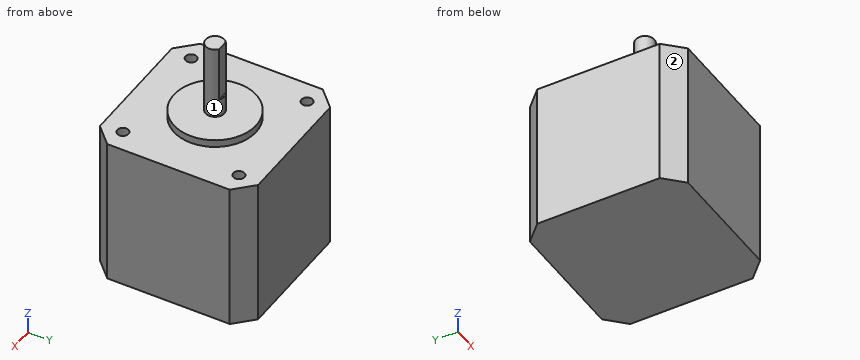
from build123d import *

# Parameters (mm, degrees)
F0_W      = 42.291
F0_H      = 42.291
F1_DEPTH  = 40.005
F2_SIZE   = 4.7752
F3_R      = 11
F4_DEPTH  = 2
F5_R      = 2.5
F6_DEPTH  = 22
F8_DEPTH  = 15
F10_D     = 3
F10_DEPTH = 4.4958
F10_TIP   = 0.9012909285


with BuildPart() as f1:
    # F0 (on Top) → F1 (new body)
    with BuildSketch(Plane.XY):
        Rectangle(F0_W, F0_H)
    extrude(amount=F1_DEPTH)

    # F2
    f2_edges = [f1.edges().sort_by_distance(p)[0] for p in [
        (21.1455, -21.1455, 20.0025),
        (21.1455, 21.1455, 20.0025),
        (-21.1455, 21.1455, 20.0025),
        (-21.1455, -21.1455, 20.0025),
    ]]
    chamfer(f2_edges, length=F2_SIZE)

    # F3 (on face) → F4 (join)
    with BuildSketch(Plane.XY.offset(40.005)):
        Circle(F3_R)
    extrude(amount=F4_DEPTH)

    # F5 (on face) → F6 (join)
    with BuildSketch(Plane.XY.offset(40.005)):
        Circle(F5_R)
    extrude(amount=F6_DEPTH)

    # F7 (on face) → F8 (cut)
    with BuildSketch(Plane.XY.offset(62.005)):
        with BuildLine():
            ThreePointArc((1.5, 2), (0.790569415, 2.3717082451), (0, 2.5))
            ThreePointArc((0, 2.5), (-0.790569415, 2.3717082451), (-1.5, 2))
            Line((-1.5, 2), (1.5, 2))
        make_face()
    extrude(amount=-F8_DEPTH, mode=Mode.SUBTRACT)

    # F10
    with Locations(Plane.XY.offset(40.005)):
        with Locations((-15.5, 15.5), (-15.5, -15.5), (15.5, -15.5), (15.5, 15.5)):
            Hole(F10_D / 2, depth=F10_DEPTH)
            with Locations((0, 0, -(F10_DEPTH + F10_TIP / 2))):  # 118° drill point
                Cone(0, F10_D / 2, F10_TIP, mode=Mode.SUBTRACT)


solid = f1.part
The model under review builds one solid part; all positions refer to its coordinate system, in mm. Face numbers are marked on the shaded views. A direction names the side the tool comes from. Round coordinates to 2 decimals unless told otherwise and drop trailing zeros. Loops run counter-clockwise (first coordinate to the right, second up) from the corner with the lowest first, then second, coordinate; pieces in that order, holes last. Notation, with made-up numbers: (47.5, -19.5) - (104.5, -19.5) arc R32 ccw to (104.5, 10.5) - close; hole circle Ø5 at (43.5, 70). An arc over 180 degrees is marked (long way). Use CSV: the item, a comma, the result in double quotes.
(1) Take a section at D-D, the plane x = 9. Give the boundary of the cut face in (y, z) (1 decimal).
Working result:
outline,"(-21.1, 0) - (21.1, 0) - (21.1, 40) - (6.3, 40) - (6.3, 42) - (-6.3, 42) - (-6.3, 40) - (-21.1, 40) - close"
(2) For line 1 (X direction, y = 15.5, z = 38.65); line 2 (X direction, y = 15, z = 36), list the stretches that pass through material, from the lowest coordinate up.
Working result:
line 1,"x = -21.15 to -17, -14 to 14, 17 to 21.15"
line 2,"x = -21.15 to -16.91, -14.09 to 14.09, 16.91 to 21.15"
(3) Take a section at A-A, the plane z = 18. Give the boundary of the cut face in (x, y), plus the area to 3 significant figures.
Working result:
outline,"(-21.15, -16.37) - (-16.37, -21.15) - (16.37, -21.15) - (21.15, -16.37) - (21.15, 16.37) - (16.37, 21.15) - (-16.37, 21.15) - (-21.15, 16.37) - close"
area,"1,740 mm^2"
(4) Take a section at C-C, the plane y = 0. Give the boundary of the cut face in (x, z) (1 decimal).
Working result:
outline,"(-21.1, 0) - (21.1, 0) - (21.1, 40) - (11, 40) - (11, 42) - (2.5, 42) - (2.5, 62) - (-2.5, 62) - (-2.5, 42) - (-11, 42) - (-11, 40) - (-21.1, 40) - close"
(5) Take a section at B-B, the plane x = 0. Give the boundary of the cut face in (y, z) (1 decimal).
Working result:
outline,"(-21.1, 0) - (21.1, 0) - (21.1, 40) - (11, 40) - (11, 42) - (2.5, 42) - (2.5, 47) - (2, 47) - (2, 62) - (-2.5, 62) - (-2.5, 42) - (-11, 42) - (-11, 40) - (-21.1, 40) - close"
(6) Clearance check with flat-ended pins moving along their axes: P1, Ø1.8, axis at x = 15.5, y = -15.5, coming from the -Z side; P2, Ø5, axis at x = 12, y = -5, coming from the +Z side (3 decimals); P3, Ø1.5, axis at x = 0.5, z = 53, coming from the +Y side; P4, Ø1.5, axis at x = 9.5, y = -10.5, coming from the +Z side (3 decimals). State where each tip first meets the part, or that it passes through.
Working result:
P1,"stops at z = 0"
P2,"stops at z = 42.005"
P3,"stops at y = 2"
P4,"stops at z = 40.005"
(7) Machinability: for the marked faces 1 and 2, which of the approach directions +Z, -Z, +X, -X, +Y, -Y give a long, thin tool a straight path to every point of the face, cutting with its end or side? Answer none if there is none.
Working result:
face 1,"+Z"
face 2,"+Z, -Z, -X, -Y"
